For this review, take the finished solid that the model builds, in its own axes (mm). Face numbers are marked on the shaded views. A direction names the side the tool comes from. Give positions to 0.01 mm unless a question says otherwise; leave off trailing zeros. Loops run counter-clockwise (first coordinate to the right, second up) from the corner with the lowest first, then second, coordinate; pieces in that order, holes last. Notation, with made-up numbers: (81, 57.25) -> (117, 57.25) arc R20 cw to (117, 77.25) -> close; hole circle Ø7 at (-14.5, 84.25). An arc over 180 degrees is marked (long way). One line per question, with ' | ' between items. Start each with the question number.
(1) Consider section C-C (z = -3.5). Write out the cut boundary in (x, y).
(2) Consider section D-D (z = -11). Write out the cut boundary in (x, y).
(3) Wall thickness on probe 1 along Y at (x, z) = (-16.5, -5.25); probe 2 along X at (y, z) = (1, -1.5); probe 3 along Y at (x, z) = (21, -7): over which ranges is each line inside the solid? List them lowest first.
(4) Tool access review of the marked faces 1, 2, 3 and 4: name each direction out of +Z, -Z, +X, -X, +Y, -Y from which nothing blocks a thin tool from reaching the whole face with its end or side.
(5) Draft analysis for pull direction X (two halves, no side actions). For the marked faces 5, 6 and 7, state which applies: +X half, -X half, draft (parallel to the pull), parting line (faces both ways), or undercut.
(6) Insertion check: P1, Ø6.5, axis at y = 2, z = -4.5, coming from the +X side; P2, Ø1.5, axis at y = 18.5, z = -10, coming from the +X side; P3, Ø4.5, axis at x = 11.5, z = -3.5, coming from the -Y side. Each pin has a flat end and moves straight along its axis. Give the tip position at first contact, or say it passes through.
(7) Consider section A-A (x = -18). Write out the cut boundary in (y, z), and give its area (3 significant figures).
(8) Consider section B-B (y = 13). Write out the cut boundary in (x, z).
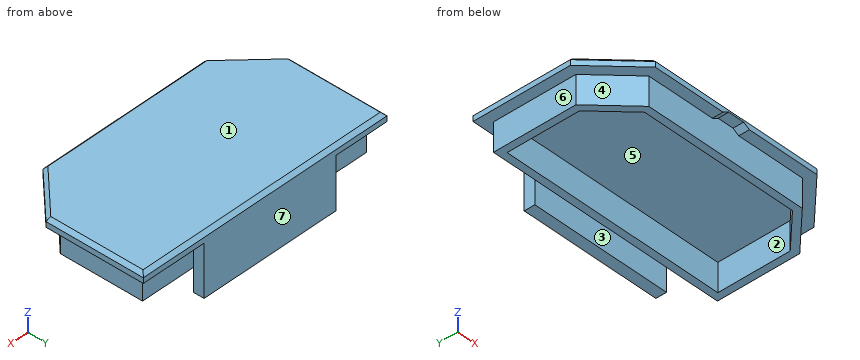
from build123d import *

# Parameters (mm, degrees)
PRESS_FIT_WALL_EXTRUDE_DEPTH = 8
MAIN_LID_EXTRUDE_DEPTH       = 2.5
MAIN_LID_CHAMFER_SIZE        = 1
MAIN_LID_TAB_CUT_DEPTH       = 3
SKETCH5_W                    = 40
SKETCH5_H                    = 3
SERVO_WALL_EXTRUDE_DEPTH     = 14.6


with BuildPart() as part:
    # Sketch2 → Press Fit Wall Extrude (new body)
    with BuildSketch(Plane.XY):
        Polygon((34, -6.3), (34, 17), (-34, 17), (-34, -6.3), (-23.3, -17), (23.3, -17), align=None)
        Polygon((32, -5.471572875), (32, 15), (-32, 15), (-32, -5.471572875), (-22.471572875, -15), (22.471572875, -15), align=None, mode=Mode.SUBTRACT)
    extrude(amount=-PRESS_FIT_WALL_EXTRUDE_DEPTH)

    # Sketch3 → Main Lid Extrude (add)
    with BuildSketch(Plane.XY):
        Polygon((24.542640687, -20), (37, -7.542640687), (37, 20), (-37, 20), (-37, -7.542640687), (-24.542640687, -20), align=None)
    extrude(amount=MAIN_LID_EXTRUDE_DEPTH)

    # Main Lid Chamfer
    main_lid_chamfer_edges = [part.edges().sort_by_distance(p)[0] for p in [
        (0, -20, 2.5),
        (30.771320344, -13.771320344, 2.5),
        (37, 6.228679656, 2.5),
        (0, 20, 2.5),
        (-37, 6.228679656, 2.5),
        (-30.771320344, -13.771320344, 2.5),
    ]]
    chamfer(main_lid_chamfer_edges, length=MAIN_LID_CHAMFER_SIZE)

    # Sketch4 → Main Lid Tab Cut (cut)
    with BuildSketch(Plane.XZ.offset(20)):
        Polygon((-4, 0), (4, 0), (2.267949192, 1), (-2.267949192, 1), align=None)
    extrude(amount=-MAIN_LID_TAB_CUT_DEPTH, mode=Mode.SUBTRACT)

    # Sketch5 → Servo Wall Extrude (add)
    with BuildSketch(Plane(origin=(0, 0, 0), x_dir=(-1, 0, 0), z_dir=(0, 0, -1))):
        with Locations((1.45, 18.5)):
            Rectangle(SKETCH5_W, SKETCH5_H)
    extrude(amount=SERVO_WALL_EXTRUDE_DEPTH)


solid = part.part
A:
1) outline: (-34, -6.3) -> (-23.3, -17) -> (23.3, -17) -> (34, -6.3) -> (34, 17) -> (18.55, 17) -> (18.55, 20) -> (-21.45, 20) -> (-21.45, 17) -> (-34, 17) -> close; hole (-32, -5.47) -> (-22.47, -15) -> (22.47, -15) -> (32, -5.47) -> (32, 15) -> (-32, 15) -> close
2) outline: (-21.45, 17) -> (18.55, 17) -> (18.55, 20) -> (-21.45, 20) -> close
3) probe 1: y = -17 to -15, 15 to 20 | probe 2: x = -34 to -32, 32 to 34 | probe 3: y = -17 to -15, 15 to 17
4) face 1: +Z, +X, -X, +Y, -Y | face 2: -Z | face 3: -Z, +X, -X, -Y | face 4: -Z, -X, -Y
5) face 5: undercut | face 6: -X half | face 7: draft
6) P1: stops at x = 34 | P2: stops at x = 18.55 | P3: stops at y = -17
7) outline: (-20, 0) -> (-17, 0) -> (-17, -8) -> (-15, -8) -> (-15, 0) -> (15, 0) -> (15, -8) -> (17, -8) -> (17, -14.6) -> (20, -14.6) -> (20, 1.5) -> (19, 2.5) -> (-19, 2.5) -> (-20, 1.5) -> close | area: 175 mm^2
8) outline: (-37, 0) -> (-34, 0) -> (-34, -8) -> (-32, -8) -> (-32, 0) -> (32, 0) -> (32, -8) -> (34, -8) -> (34, 0) -> (37, 0) -> (37, 1.5) -> (36, 2.5) -> (-36, 2.5) -> (-37, 1.5) -> close
